from build123d import *
from build123d.topology import SkipClean

# Parameters (mm, degrees)
SKETCH1_R           = 13.25
SKETCH1_R_2         = 10.5
BOSS_EXTRUDE1_DEPTH = 6.5
BOSS_EXTRUDE2_START = 1.3
SKETCH1_3_R         = 13.25
SKETCH1_3_R_2       = 10.5
BOSS_EXTRUDE2_DEPTH = 1.3


with BuildPart() as part:
    # Sketch1 → Boss-Extrude1 (new body)
    # profile 1 of 4: a face of its own
    with BuildSketch(Plane(origin=(0, 0, 0), x_dir=(1, 0, 0), z_dir=(0, 1, 0))):
        Circle(SKETCH1_R)
        with Locations(Location((0, 0, 0), (0, 0, 270))):
            Circle(SKETCH1_R_2, mode=Mode.SUBTRACT)
    # profile 2 of 4: a face of its own
    with BuildSketch(Plane(origin=(0, 0, 0), x_dir=(1, 0, 0), z_dir=(0, 1, 0))):
        with BuildLine():
            ThreePointArc((10.343362597, -8.281144256), (0, -13.25), (-10.343362597, -8.281144256))
            Line((-10.343362597, -8.281144256), (-11.437342964, -8.912754116))
            ThreePointArc((-11.437342964, -8.912754116), (0, -14.5), (11.437342964, -8.912754116))
            Line((11.437342964, -8.912754116), (10.343362597, -8.281144256))
        make_face()
    # profile 3 of 4: a face of its own
    with BuildSketch(Plane(origin=(0, 0, 0), x_dir=(1, 0, 0), z_dir=(0, 1, 0))):
        with BuildLine():
            Line((2, 14.361406616), (2, 13.098186897))
            ThreePointArc((2, 13.098186897), (10.051430246, 8.633148325), (13.25, 0))
            ThreePointArc((13.25, 0), (13.0213681, -2.450810641), (12.343362597, -4.817042641))
            Line((12.343362597, -4.817042641), (13.437342964, -5.448652501))
            ThreePointArc((13.437342964, -5.448652501), (14.231856396, -2.77565551), (14.5, 0))
            ThreePointArc((14.5, 0), (10.937321427, 9.519716382), (2, 14.361406616))
        make_face()
    # profile 4 of 4: a face of its own
    with BuildSketch(Plane(origin=(0, 0, 0), x_dir=(1, 0, 0), z_dir=(0, 1, 0))):
        with BuildLine():
            ThreePointArc((-12.343362597, -4.817042641), (-11.4748366, 6.625), (-2, 13.098186897))
            Line((-2, 13.098186897), (-2, 14.361406616))
            ThreePointArc((-2, 14.361406616), (-12.557368355, 7.25), (-13.437342964, -5.448652501))
            Line((-13.437342964, -5.448652501), (-12.343362597, -4.817042641))
        make_face()
    extrude(amount=-BOSS_EXTRUDE1_DEPTH)

    # Sketch1_3 → Boss-Extrude2 (add)
    # profile 1 of 7: a face of its own
    with SkipClean():  # the faces are left unmerged after this step: merging them gives an invalid solid
        with BuildSketch(Plane(origin=(0, 0, 0), x_dir=(1, 0, 0), z_dir=(0, 1, 0)).offset(BOSS_EXTRUDE2_START)):
            with BuildLine():
                ThreePointArc((-12.343362597, -4.817042641), (-11.4748366, 6.625), (-2, 13.098186897))
                Line((-2, 13.098186897), (-2, 14.361406616))
                ThreePointArc((-2, 14.361406616), (-12.557368355, 7.25), (-13.437342964, -5.448652501))
                Line((-13.437342964, -5.448652501), (-12.343362597, -4.817042641))
            make_face()
        # profile 2 of 7: a face of its own
        with BuildSketch(Plane(origin=(0, 0, 0), x_dir=(1, 0, 0), z_dir=(0, 1, 0)).offset(BOSS_EXTRUDE2_START)):
            Circle(SKETCH1_3_R)
            with Locations(Location((0, 0, 0), (0, 0, 270))):
                Circle(SKETCH1_3_R_2, mode=Mode.SUBTRACT)
        # profile 3 of 7: a face of its own
        with BuildSketch(Plane(origin=(0, 0, 0), x_dir=(1, 0, 0), z_dir=(0, 1, 0)).offset(BOSS_EXTRUDE2_START)):
            with BuildLine():
                Line((13.437342964, -5.448652501), (12.343362597, -4.817042641))
                ThreePointArc((12.343362597, -4.817042641), (11.4748366, -6.625), (10.343362597, -8.281144256))
                Line((10.343362597, -8.281144256), (11.437342964, -8.912754116))
                ThreePointArc((11.437342964, -8.912754116), (12.557368355, -7.25), (13.437342964, -5.448652501))
            make_face()
        # profile 4 of 7: a face of its own
        with BuildSketch(Plane(origin=(0, 0, 0), x_dir=(1, 0, 0), z_dir=(0, 1, 0)).offset(BOSS_EXTRUDE2_START)):
            with BuildLine():
                ThreePointArc((10.343362597, -8.281144256), (0, -13.25), (-10.343362597, -8.281144256))
                Line((-10.343362597, -8.281144256), (-11.437342964, -8.912754116))
                ThreePointArc((-11.437342964, -8.912754116), (0, -14.5), (11.437342964, -8.912754116))
                Line((11.437342964, -8.912754116), (10.343362597, -8.281144256))
            make_face()
        # profile 5 of 7: a face of its own
        with BuildSketch(Plane(origin=(0, 0, 0), x_dir=(1, 0, 0), z_dir=(0, 1, 0)).offset(BOSS_EXTRUDE2_START)):
            with BuildLine():
                ThreePointArc((-10.343362597, -8.281144256), (-11.4748366, -6.625), (-12.343362597, -4.817042641))
                Line((-12.343362597, -4.817042641), (-13.437342964, -5.448652501))
                ThreePointArc((-13.437342964, -5.448652501), (-12.557368355, -7.25), (-11.437342964, -8.912754116))
                Line((-11.437342964, -8.912754116), (-10.343362597, -8.281144256))
            make_face()
        # profile 6 of 7: a face of its own
        with BuildSketch(Plane(origin=(0, 0, 0), x_dir=(1, 0, 0), z_dir=(0, 1, 0)).offset(BOSS_EXTRUDE2_START)):
            with BuildLine():
                Line((2, 14.361406616), (2, 13.098186897))
                ThreePointArc((2, 13.098186897), (10.051430246, 8.633148325), (13.25, 0))
                ThreePointArc((13.25, 0), (13.0213681, -2.450810641), (12.343362597, -4.817042641))
                Line((12.343362597, -4.817042641), (13.437342964, -5.448652501))
                ThreePointArc((13.437342964, -5.448652501), (14.231856396, -2.77565551), (14.5, 0))
                ThreePointArc((14.5, 0), (10.937321427, 9.519716382), (2, 14.361406616))
            make_face()
        # profile 7 of 7: a face of its own
        with BuildSketch(Plane(origin=(0, 0, 0), x_dir=(1, 0, 0), z_dir=(0, 1, 0)).offset(BOSS_EXTRUDE2_START)):
            with BuildLine():
                Line((-2, 14.361406616), (-2, 13.098186897))
                ThreePointArc((-2, 13.098186897), (0, 13.25), (2, 13.098186897))
                Line((2, 13.098186897), (2, 14.361406616))
                ThreePointArc((2, 14.361406616), (0, 14.5), (-2, 14.361406616))
            make_face()
        extrude(amount=-BOSS_EXTRUDE2_DEPTH)


solid = part.part
Geometry: final body of the model. Coordinates: model frame, mm. A direction names the side the tool comes from. Round coordinates to 2 decimals unless told otherwise and drop trailing zeros. Loops run counter-clockwise (first coordinate to the right, second up) from the corner with the lowest first, then second, coordinate; pieces in that order, holes last.
Q1. Section A-A on x = 0. Return loops of the section in (y, z).
Q2. Pin query (flat end, axial travel): P1, Ø1.1, axis at x = 0.5, z = -14, coming from the -Y side; P2, Ø17, axis at x = 0, z = 0, coming from the +Y side; P3, Ø3, axis at y = -1, z = 2, coming from the -X side; P4, Ø0.6, axis at y = -4, z = -13.5, coming from the +X side. Return the tip coordinate at first contact, or that it passes through.
Q3. Access query for faces 4 (the flat face through (12.883, -3.204, 5.128)), 5 (the flat face through (0, 0, -14)), 6 (the cylindrical face through (-11.49, -3.2, 6.6)), 7 (the flat face through (10.898, -3.204, 8.601)). Directions: +Z, -Z, +X, -X, +Y, -Y. A direction counts if a zero-diameter tool reaches every point of the face in a straight line with its end or side. Return the directions, or none.
Q4. Material intervals for L1, parallel to Z at x = -8.25, y = -5.25; L2, parallel to X at y = 0.5, z = -1.5; L3, parallel to Z at x = 1.25, y = -5.75, sorted ascending.
Q5. Section C-C on y = -2.75. Return loops of the section in (x, z), plus the area to 3 significant figures.
Q6. Section B-B on z = 3.75. Return loops of the section in (x, y).
Q7. Pull-direction query (Z, two-part tool) for faces 1 (the flat face through (-10.88, -3.2, 8.59)), 2 (the flat face through (-2, -3, -14)), 3 (the flat face through (-12.9, -3.2, 5.14)); classes: released by +Z, released by -Z, zero draft, split by the parting line, or undercut.
Q8. Section D-D on z = 0.75. Return loops of the section in (x, y).
Evaluation:
1. outline: (-6.5, -13.25) - (0, -13.25) - (0, -14.5) - (1.3, -14.5) - (1.3, -10.5) - (-6.5, -10.5) - close; (-6.5, 10.5) - (1.3, 10.5) - (1.3, 14.5) - (-6.5, 14.5) - close
2. P1: stops at y = 0
2. P2: passes through
2. P3: stops at x = -14.49
2. P4: stops at x = 6
3. face 4: +Z, -Y
3. face 5: -Z, -Y
3. face 6: -Y
3. face 7: +X, -Y
4. L1: z = -11.92 to -6.5, 6.5 to 11.92
4. L2: x = -14.42 to -10.39, 10.39 to 14.42
4. L3: z = -13.19 to -10.43, 10.43 to 14.45
5. outline: (-13.44, 5.45) arc R14.5 ccw to (-2, -14.36) - (-2, -13.1) arc R13.25 ccw to (2, -13.1) - (2, -14.36) arc R14.5 ccw to (13.44, 5.45) - (12.34, 4.82) arc R13.25 ccw to (10.34, 8.28) - (11.44, 8.91) arc R14.5 ccw to (-11.44, 8.91) - (-10.34, 8.28) arc R13.25 ccw to (-12.34, 4.82) - close; hole circle Ø21 at (0, 0)
5. area: 299 mm2
6. outline: (-14.01, -6.5) - (-9.81, -6.5) - (-9.81, 1.3) - (-14.01, 1.3) - close; (9.81, -6.5) - (14.01, -6.5) - (14.01, 1.3) - (9.81, 1.3) - close
7. face 1: undercut
7. face 2: zero draft
7. face 3: released by +Z
8. outline: (-14.48, -6.5) - (-10.47, -6.5) - (-10.47, 1.3) - (-14.48, 1.3) - close; (10.47, -6.5) - (14.48, -6.5) - (14.48, 1.3) - (10.47, 1.3) - close
